Part model, mm, in its own coordinate system. A direction names the side the tool comes from. Give positions to 0.01 mm unless a question says otherwise; leave off trailing zeros. Order: outer loops, then holes, each group sorted by start corner. A loop starts at its lowest first (then second) coordinate and runs counter-clockwise, first axis right, second up. Notation, with made-up numbers: M 29.25,26.5 L 69.25,26.5 A21 ccw 69.25,54.5 Z; hole C 67,88 d3. An arc over 180 degrees is marked long. Return JSON: item names as keys, results as strings.
from build123d import *

# Parameters (mm, degrees)
SKETCH001_W     = 10.6
SKETCH001_H     = 6
POCKET_DEPTH    = 3
SKETCH002_R     = 1.75
POCKET001_DEPTH = 22


with BuildPart() as part:
    # Sketch → Revolution (revolve)
    with BuildSketch(Plane.XY):
        with BuildLine():
            Line((7.25, 17.75), (7.25, 0))
            Line((7.25, 0), (0, 0))
            Line((0, 0), (0, 25))
            ThreePointArc((7.25, 17.75), (5.126524, 22.876524), (0, 25))
        make_face()
    revolve(axis=Axis((0, 0, 0), (0, 1, 0)))

    # Sketch001 (on DatumPlane) → Pocket (cut)
    with BuildSketch(Plane.XZ.offset(-5)):
        Rectangle(SKETCH001_W, SKETCH001_H)
    extrude(amount=-POCKET_DEPTH, mode=Mode.SUBTRACT)

    # Sketch002 → Pocket001 (cut)
    with BuildSketch(Plane.XZ):
        Circle(SKETCH002_R)
    extrude(amount=-POCKET001_DEPTH, mode=Mode.SUBTRACT)


solid = part.part
Q1. Probe line 1 along Z through (x, y) = (0, 11); line 2 along Y through (x, z) = (-2.25, 0.75); line 3 along Y through (x, z) = (-5, 1). List the from-to ranges inside material, lowest first.
Established:
{"line 1": "z = -7.25 to -1.75, 1.75 to 7.25", "line 2": "y = 0 to 5, 8 to 24.6", "line 3": "y = 0 to 5, 8 to 22.9"}
Q2. Two-plate mould, pull along Z, no slides. Class faces 3 (the cylindrical face through (3.35, 8.75, 6.43)), 4 (the flat face through (2, 0, 2)), 5 (the cylindrical face through (1.617, 14.902, -0.67)): +Z half, -Z half, draft (parallel to the pull), parting line (faces both ways), or undercut.
Established:
{"face 3": "parting line", "face 4": "draft", "face 5": "undercut"}
Q3. Band-saw the part on A-A (y = 2.5). Give the cut face in (x, z), then the cut area to 3 significant figures.
Established:
{"outline": "C 0,0 d14.5; hole C 0,0 d3.5", "area": "156 mm²"}
Q4. Pin check, flat tips, straight feed: pin 1 (2.5 mm diameter, centred on y = 6.5, z = -1.5, fed in from +X); pin 2 (3 mm diameter, centred on y = 20.5, z = -2.5, fed in from -X); pin 3 (1.8 mm diameter, centred on x = 0, z = -0.5, fed in from -Y). Stop position of each tip, or through.
Established:
{"pin 1": "stops at x = 7.25", "pin 2": "stops at x = -6.9", "pin 3": "stops at y = 22"}
Q5. 3-axis set-ups, long thin cutter, end or side, ignore diameter. For faces 1 (the flat face through (5.3, 6, 0)), 2 (the cylindrical face through (1.617, 2.465, -0.67)): which of +Z, -Z, +X, -X, +Y, -Y reach the whole face in a straight line?
Established:
{"face 1": "none", "face 2": "-Y"}
